```python
from build123d import *

# Parameters (mm, degrees)
Y_KSEKLIK_EKSTR_ZYON2_DEPTH = 160
RADYUS1_R                   = 0.8


with BuildPart() as part:
    # Çizim3 → Yükseklik-Ekstrüzyon2 (new body, symmetric)
    with BuildSketch(Plane.XY):
        with BuildLine():
            Line((1, 0), (6.1, 0))
            Line((6.1, 0), (6.1, 0.5))
            Line((6.1, 0.5), (6.85, 0.5))
            Line((6.85, 0.5), (6.85, 1.4))
            Line((6.85, 1.4), (4.321320344, 1.4))
            ThreePointArc((4.321320344, 1.4), (3.582216718, 1.893853254), (3.755634919, 2.765685425))
            Line((3.755634919, 2.765685425), (7.638403375, 6.648453882))
            ThreePointArc((7.638403375, 6.648453882), (10, 5.9), (12.361596625, 6.648453882))
            Line((12.361596625, 6.648453882), (16.244365081, 2.765685425))
            ThreePointArc((16.244365081, 2.765685425), (16.417783282, 1.893853254), (15.678679656, 1.4))
            Line((15.678679656, 1.4), (13.15, 1.4))
            Line((13.15, 1.4), (13.15, 0.5))
            Line((13.15, 0.5), (13.9, 0.5))
            Line((13.9, 0.5), (13.9, 0))
            Line((13.9, 0), (26.1, 0))
            Line((26.1, 0), (26.1, 0.5))
            Line((26.1, 0.5), (26.85, 0.5))
            Line((26.85, 0.5), (26.85, 1.4))
            Line((26.85, 1.4), (24.321320344, 1.4))
            ThreePointArc((24.321320344, 1.4), (23.582216718, 1.893853254), (23.755634919, 2.765685425))
            Line((23.755634919, 2.765685425), (27.638403375, 6.648453882))
            ThreePointArc((27.638403375, 6.648453882), (30, 5.9), (32.361596625, 6.648453882))
            Line((32.361596625, 6.648453882), (36.244365081, 2.765685425))
            ThreePointArc((36.244365081, 2.765685425), (36.417783282, 1.893853254), (35.678679656, 1.4))
            Line((35.678679656, 1.4), (33.15, 1.4))
            Line((33.15, 1.4), (33.15, 0.5))
            Line((33.15, 0.5), (33.9, 0.5))
            Line((33.9, 0.5), (33.9, 0))
            Line((33.9, 0), (39, 0))
            ThreePointArc((39, 0), (39.707106781, 0.292893219), (40, 1))
            Line((40, 1), (40, 6.1))
            Line((40, 6.1), (39.5, 6.1))
            Line((39.5, 6.1), (39.5, 6.85))
            Line((39.5, 6.85), (38.6, 6.85))
            Line((38.6, 6.85), (38.6, 4.321320344))
            ThreePointArc((38.6, 4.321320344), (38.106146746, 3.582216718), (37.234314575, 3.755634919))
            Line((37.234314575, 3.755634919), (33.351546118, 7.638403375))
            ThreePointArc((33.351546118, 7.638403375), (34.1, 10), (33.351546118, 12.361596625))
            Line((33.351546118, 12.361596625), (37.234314575, 16.244365081))
            ThreePointArc((37.234314575, 16.244365081), (38.106146746, 16.417783282), (38.6, 15.678679656))
            Line((38.6, 15.678679656), (38.6, 13.15))
            Line((38.6, 13.15), (39.5, 13.15))
            Line((39.5, 13.15), (39.5, 13.9))
            Line((39.5, 13.9), (40, 13.9))
            Line((40, 13.9), (40, 19))
            ThreePointArc((40, 19), (39.707106781, 19.707106781), (39, 20))
            Line((39, 20), (33.9, 20))
            Line((33.9, 20), (33.9, 19.5))
            Line((33.9, 19.5), (33.15, 19.5))
            Line((33.15, 19.5), (33.15, 18.6))
            Line((33.15, 18.6), (35.678679656, 18.6))
            ThreePointArc((35.678679656, 18.6), (36.417783282, 18.106146746), (36.244365081, 17.234314575))
            Line((36.244365081, 17.234314575), (32.361596625, 13.351546118))
            ThreePointArc((32.361596625, 13.351546118), (30, 14.1), (27.638403375, 13.351546118))
            Line((27.638403375, 13.351546118), (23.755634919, 17.234314575))
            ThreePointArc((23.755634919, 17.234314575), (23.582216718, 18.106146746), (24.321320344, 18.6))
            Line((24.321320344, 18.6), (26.85, 18.6))
            Line((26.85, 18.6), (26.85, 19.5))
            Line((26.85, 19.5), (26.1, 19.5))
            Line((26.1, 19.5), (26.1, 20))
            Line((26.1, 20), (13.9, 20))
            Line((13.9, 20), (13.9, 19.5))
            Line((13.9, 19.5), (13.15, 19.5))
            Line((13.15, 19.5), (13.15, 18.6))
            Line((13.15, 18.6), (15.678679656, 18.6))
            ThreePointArc((15.678679656, 18.6), (16.417783282, 18.106146746), (16.244365081, 17.234314575))
            Line((16.244365081, 17.234314575), (12.361596625, 13.351546118))
            ThreePointArc((12.361596625, 13.351546118), (10, 14.1), (7.638403375, 13.351546118))
            Line((7.638403375, 13.351546118), (3.755634919, 17.234314575))
            ThreePointArc((3.755634919, 17.234314575), (3.582216718, 18.106146746), (4.321320344, 18.6))
            Line((4.321320344, 18.6), (6.85, 18.6))
            Line((6.85, 18.6), (6.85, 19.5))
            Line((6.85, 19.5), (6.1, 19.5))
            Line((6.1, 19.5), (6.1, 20))
            Line((6.1, 20), (1, 20))
            ThreePointArc((1, 20), (0.292893219, 19.707106781), (0, 19))
            Line((0, 19), (0, 13.9))
            Line((0, 13.9), (0.5, 13.9))
            Line((0.5, 13.9), (0.5, 13.15))
            Line((0.5, 13.15), (1.4, 13.15))
            Line((1.4, 13.15), (1.4, 15.678679656))
            ThreePointArc((1.4, 15.678679656), (1.893853254, 16.417783282), (2.765685425, 16.244365081))
            Line((2.765685425, 16.244365081), (6.648453882, 12.361596625))
            ThreePointArc((6.648453882, 12.361596625), (5.9, 10), (6.648453882, 7.638403375))
            Line((6.648453882, 7.638403375), (2.765685425, 3.755634919))
            ThreePointArc((2.765685425, 3.755634919), (1.893853254, 3.582216718), (1.4, 4.321320344))
            Line((1.4, 4.321320344), (1.4, 6.85))
            Line((1.4, 6.85), (0.5, 6.85))
            Line((0.5, 6.85), (0.5, 6.1))
            Line((0.5, 6.1), (0, 6.1))
            Line((0, 6.1), (0, 1))
            ThreePointArc((0, 1), (0.292893219, 0.292893219), (1, 0))
        make_face()
        with BuildLine():
            Line((21.210320913, 18.6), (18.789679087, 18.6))
            ThreePointArc((18.789679087, 18.6), (18.223993662, 18.365685425), (17.989679087, 17.8))
            Line((17.989679087, 17.8), (17.989679087, 17.331100443))
            ThreePointArc((17.989679087, 17.331100443), (17.928782713, 17.024953697), (17.755364512, 16.765415018))
            Line((17.755364512, 16.765415018), (13.351546118, 12.361596625))
            ThreePointArc((13.351546118, 12.361596625), (14.1, 10), (13.351546118, 7.638403375))
            Line((13.351546118, 7.638403375), (17.755364512, 3.234584982))
            ThreePointArc((17.755364512, 3.234584982), (17.928782713, 2.975046303), (17.989679087, 2.668899557))
            Line((17.989679087, 2.668899557), (17.989679087, 2.2))
            ThreePointArc((17.989679087, 2.2), (18.223993662, 1.634314575), (18.789679087, 1.4))
            Line((18.789679087, 1.4), (21.210320913, 1.4))
            ThreePointArc((21.210320913, 1.4), (21.776006338, 1.634314575), (22.010320913, 2.2))
            Line((22.010320913, 2.2), (22.010320913, 2.668899557))
            ThreePointArc((22.010320913, 2.668899557), (22.071217287, 2.975046303), (22.244635488, 3.234584982))
            Line((22.244635488, 3.234584982), (26.648453882, 7.638403375))
            ThreePointArc((26.648453882, 7.638403375), (25.9, 10), (26.648453882, 12.361596625))
            Line((26.648453882, 12.361596625), (22.244635488, 16.765415018))
            ThreePointArc((22.244635488, 16.765415018), (22.071217287, 17.024953697), (22.010320913, 17.331100443))
            Line((22.010320913, 17.331100443), (22.010320913, 17.8))
            ThreePointArc((22.010320913, 17.8), (21.776006338, 18.365685425), (21.210320913, 18.6))
        make_face(mode=Mode.SUBTRACT)
        with BuildLine():
            Line((8.201142588, 12.443783276), (8.552743846, 12.092182018))
            ThreePointArc((8.552743846, 12.092182018), (10, 12.543968548), (11.447256154, 12.092182018))
            Line((11.447256154, 12.092182018), (11.798857412, 12.443783276))
            ThreePointArc((11.798857412, 12.443783276), (12.443783276, 12.443783276), (12.443783276, 11.798857412))
            Line((12.443783276, 11.798857412), (12.092182018, 11.447256154))
            ThreePointArc((12.092182018, 11.447256154), (12.543968548, 10), (12.092182018, 8.552743846))
            Line((12.092182018, 8.552743846), (12.443783276, 8.201142588))
            ThreePointArc((12.443783276, 8.201142588), (12.443783276, 7.556216724), (11.798857412, 7.556216724))
            Line((11.798857412, 7.556216724), (11.447256154, 7.907817982))
            ThreePointArc((11.447256154, 7.907817982), (10, 7.456031452), (8.552743846, 7.907817982))
            Line((8.552743846, 7.907817982), (8.201142588, 7.556216724))
            ThreePointArc((8.201142588, 7.556216724), (7.556216724, 7.556216724), (7.556216724, 8.201142588))
            Line((7.556216724, 8.201142588), (7.907817982, 8.552743846))
            ThreePointArc((7.907817982, 8.552743846), (7.456031452, 10), (7.907817982, 11.447256154))
            Line((7.907817982, 11.447256154), (7.556216724, 11.798857412))
            ThreePointArc((7.556216724, 11.798857412), (7.556216724, 12.443783276), (8.201142588, 12.443783276))
        make_face(mode=Mode.SUBTRACT)
        with BuildLine():
            Line((27.907817982, 11.447256154), (27.556216724, 11.798857412))
            ThreePointArc((27.556216724, 11.798857412), (27.556216724, 12.443783276), (28.201142588, 12.443783276))
            Line((28.201142588, 12.443783276), (28.552743846, 12.092182018))
            ThreePointArc((28.552743846, 12.092182018), (30, 12.543968548), (31.447256154, 12.092182018))
            Line((31.447256154, 12.092182018), (31.798857412, 12.443783276))
            ThreePointArc((31.798857412, 12.443783276), (32.443783276, 12.443783276), (32.443783276, 11.798857412))
            Line((32.443783276, 11.798857412), (32.092182018, 11.447256154))
            ThreePointArc((32.092182018, 11.447256154), (32.543968548, 10), (32.092182018, 8.552743846))
            Line((32.092182018, 8.552743846), (32.443783276, 8.201142588))
            ThreePointArc((32.443783276, 8.201142588), (32.443783276, 7.556216724), (31.798857412, 7.556216724))
            Line((31.798857412, 7.556216724), (31.447256154, 7.907817982))
            ThreePointArc((31.447256154, 7.907817982), (30, 7.456031452), (28.552743846, 7.907817982))
            Line((28.552743846, 7.907817982), (28.201142588, 7.556216724))
            ThreePointArc((28.201142588, 7.556216724), (27.556216724, 7.556216724), (27.556216724, 8.201142588))
            Line((27.556216724, 8.201142588), (27.907817982, 8.552743846))
            ThreePointArc((27.907817982, 8.552743846), (27.456031452, 10), (27.907817982, 11.447256154))
        make_face(mode=Mode.SUBTRACT)
    extrude(amount=Y_KSEKLIK_EKSTR_ZYON2_DEPTH, both=True)

    # Radyus1
    radyus1_edges = [part.edges().sort_by_distance(p)[0] for p in [
        (6.648453882, 7.638403375, 0),
        (6.648453882, 12.361596625, 0),
        (33.351546118, 12.361596625, 0),
        (33.351546118, 7.638403375, 0),
        (13.351546118, 12.361596625, 0),
        (13.351546118, 7.638403375, 0),
        (26.648453882, 7.638403375, 0),
        (26.648453882, 12.361596625, 0),
    ]]
    fillet(radyus1_edges, radius=RADYUS1_R)


solid = part.part
```
Can you work these out from the model? Positions are in its coordinate system, mm. Give positions to 0.01 mm unless a question says otherwise; leave off trailing zeros. Write item = value, one per line. Start each with the question number.
1. For pin 1 (6 mm diameter, centred on y = 13, z = -82, fed in from +X); pin 2 (1.5 mm diameter, centred on x = 27.5, z = 24.5, fed in from +Y); pin 3 (0.6 mm diameter, centred on y = 0, z = -1, fed in from +X); pin 4 (5 mm diameter, centred on y = 9, z = 72.5, fed in from +X), each with a flat end and sliding along its axis, tell me the tip position at first contact or that it passes through.
2. Please list where these lines run through material, in increasing order: line 1 (X direction, y = 11.75, z = -21.5); line 2 (X direction, y = 18, z = -81.5); line 3 (X direction, y = 14.75, z = -87).
3. Imagine slicing it at A-A (z = 16.5). Count the separate pieces of the cut face and the enclosed holes in it, and give its area (3 significant figures).
4. Thinking about a two-plate mould opening in Z: for faces 1 (the face through (15, 5, 160)), 2 (the face through (15, 5, -160)), 3 (the face through (4, 20, 2)), which applies, released by +Z, released by -Z, zero draft, split by the parting line, or undercut?
Worked answers:
q1.pin_1 = 40
q1.pin_2 = 19.5
q1.pin_3 = 39.71
q1.pin_4 = 39.5
q2.line_1 = 6.29 to 7.61, 12.39 to 13.71, 26.29 to 27.61, 32.39 to 33.71
q2.line_2 = 0 to 3.55, 16.45 to 18.02, 21.98 to 23.55, 36.45 to 40
q2.line_3 = 0 to 1.4, 4.26 to 6.24, 13.76 to 15.74, 24.26 to 26.24, 33.76 to 35.74, 38.6 to 40
q3.separate_pieces = 1
q3.enclosed_holes = 3
q3.area = 255 mm2
q4.face_1 = released by +Z
q4.face_2 = released by -Z
q4.face_3 = zero draft
